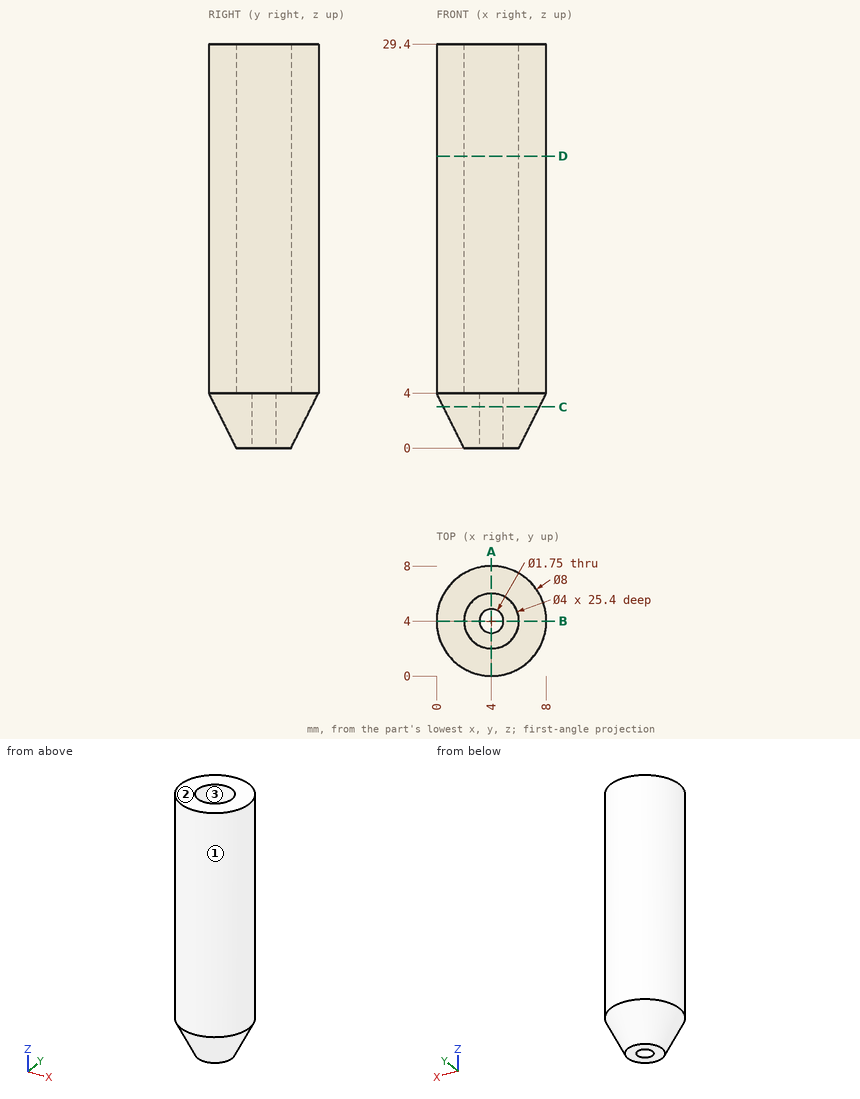
The figure shows three views and two pictorial views of one solid part (mm, origin at its lowest corner). Answer the questions. Coordinates: 2 decimals unless noted, no trailing zeros. Loops run counter-clockwise (first coordinate to the right, second up) from the corner with the lowest first, then second, coordinate; pieces in that order, holes last.
(1) The part is cut by section C-C (z = 3). Determine the outline of the cut face in (x, y) (3 decimals), and give its area (3 significant figures).
Solution:
outline: circle Ø7 at (4, 4); hole circle Ø1.75 at (4, 4)
area: 36.1 mm2
(2) Consider line 1 along Y through (x, z) = (4, 12.5); line 2 along Y through (x, z) = (4, 1.25) (3 decimals); line 3 along Z through (x, y) = (1.25, 2.5). Determine where each line is inside the solid, lowest interval first.
Solution:
line 1: y = 0 to 2, 6 to 8
line 2: y = 1.375 to 3.125, 4.875 to 6.625
line 3: z = 2.26 to 29.4
(3) A flat-ended cylindrical pin translates along its axis: pin 1 Ø4 at (x, z) = (4.5, 13) entering from +Y. Find the tip coordinate at first contact, or state that the pin passes through.
Solution:
pin 1: stops at y = 8
(4) The part is cut by section D-D (z = 21.25). Determine the outline of the cut face in (x, y).
Solution:
outline: circle Ø8 at (4, 4); hole circle Ø4 at (4, 4)
(5) The part is cut by section A-A (x = 4). Determine the outline of the cut face in (y, z) (3 decimals).
Solution:
outline: (0, 4) - (2, 0) - (3.125, 0) - (3.125, 4) - (2, 4) - (2, 29.4) - (0, 29.4) - close; (4.875, 0) - (6, 0) - (8, 4) - (8, 29.4) - (6, 29.4) - (6, 4) - (4.875, 4) - close
(6) The mould has two halves that part along Y. Classify the marked faces 1, 2 and 3: released by +Y, released by -Y, zero draft, split by the parting line, or undercut.
Solution:
face 1: split by the parting line
face 2: zero draft
face 3: undercut
